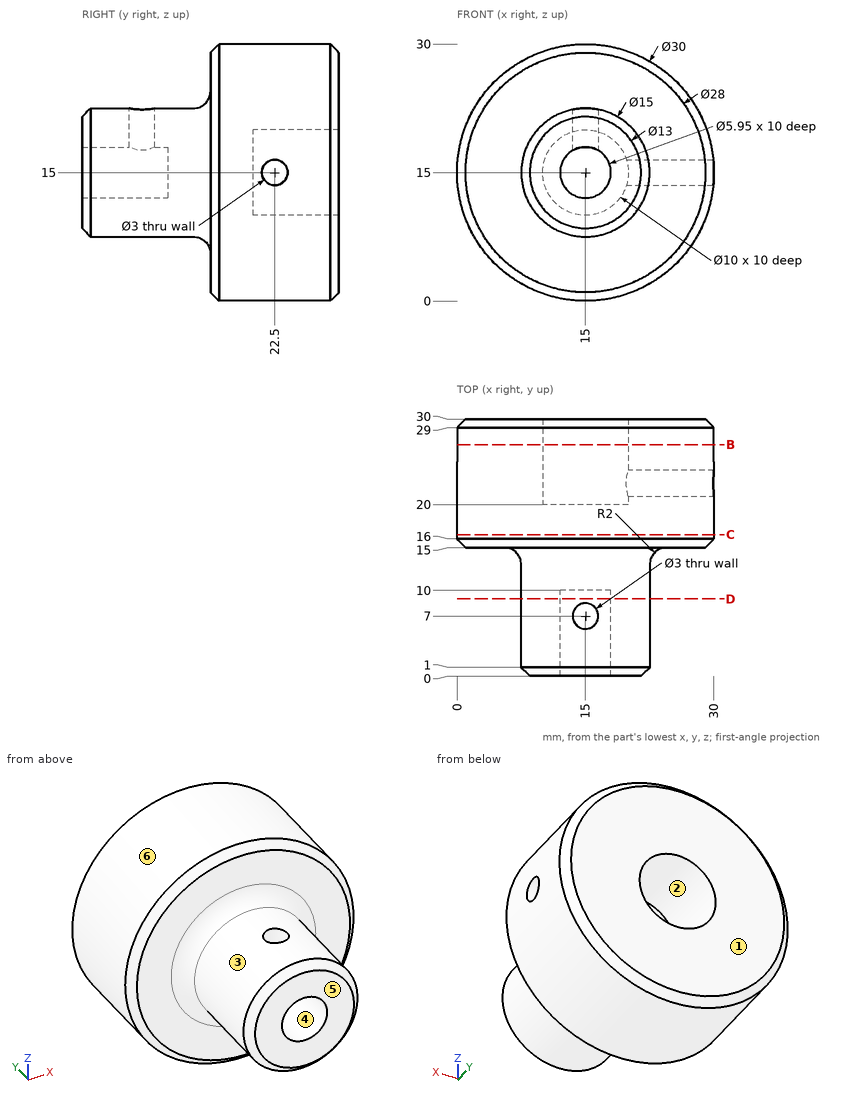
Check sheet for the drawn part. Datum: minimum x, y, z corner. Units: mm. A direction names the side the tool comes from. Give positions to 0.01 mm unless a question says otherwise; leave off trailing zeros. Loops run counter-clockwise (first coordinate to the right, second up) from the corner with the lowest first, then second, coordinate; pieces in that order, holes last. Notation, with made-up numbers: M -9,-18.5 L 9,-18.5 A27 cw 9,1.5 Z; hole C -7,84 d7. An arc over 180 degrees is marked long. Answer as CSV lines item,"result".
Item 1: Scan lines: L1, parallel to Y at x = 15, z = 19; L2, parallel to Z at x = 15, y = 3.5 (3 decimals); L3, parallel to Y at x = 12, z = 4.5. Record each from-to range of solid material in increasing order.
Reply:
L1,"0 to 5.5, 8.5 to 20"
L2,"7.5 to 12.025, 17.975 to 22.5"
L3,"15 to 30"
Item 2: Sectioned sample at C-C, the plane y = 16.5. Enter the section's corners in (x, z).
Reply:
outline,"C 15,15 d30"
Item 3: Sectioned sample at B-B, the plane y = 27. Enter the section's corners in (x, z).
Reply:
outline,"C 15,15 d30; hole C 15,15 d10"
Item 4: Draft check along Z on the marked faces 4, 5 and 6. Enter one of: pulls with the +Z half, pulls with the -Z half, needs draft (parallel to the pull), parting line crosses it, or undercut.
Reply:
face 4,"undercut"
face 5,"needs draft"
face 6,"parting line crosses it"
Item 5: Set-up check for the marked faces 1, 2 and 3: record each of +Z, -Z, +X, -X, +Y, -Y from which the full face is reachable in a straight line by a thin tool's end or side.
Reply:
face 1,"+Z, -Z, +X, -X, +Y"
face 2,"+Y"
face 3,"-Y"
Item 6: Depth check by flat-ended pin: pin 1 Ø12 at (y, z) = (17.5, 24) entering from +X; pin 2 Ø1 at (x, y) = (20, 23.5) entering from +Z; pin 3 Ø1.8 at (x, z) = (14, 15) entering from -Y; pin 4 Ø11 at (x, z) = (17, 14) entering from +Y. Enter the tip coordinate at first touch or a pass-through.
Reply:
pin 1,"x = 29.7"
pin 2,"z = 29.31"
pin 3,"y = 10"
pin 4,"y = 30"
Item 7: Sectioned sample at D-D, the plane y = 9. Enter the section's corners in (x, z) (3 decimals), then the cut area to 3 significant figures.
Reply:
outline,"C 15,15 d15; hole C 15,15 d5.95"
area,"149 mm^2"
